Job drawing, mm, ordinate dimensions from the low corner. One solid piece. A direction names the side the tool comes from. Round coordinates to 2 decimals unless told otherwise and drop trailing zeros. Loops run counter-clockwise (first coordinate to the right, second up) from the corner with the lowest first, then second, coordinate; pieces in that order, holes last. Notation, with made-up numbers: M 55,-38 L 106,-38 A20 ccw 106,-12 Z; hole C 62.25,63 d4. An arc over 180 degrees is marked long. Put each result on its own line as item: value. Start each with the question number.
1) Slice it at C-C on y = 45. Give the cut face in (x, z) (1 decimal).
2) Slice it at D-D on x = 25.5. Give the cut face in (y, z).
3) Slice it at B-B on z = 28.5. Give the cut face in (x, y).
4) Probe line 1 along X through (y, z) = (35.5, 33); line 2 along Y through (x, z) = (3, 19); line 3 along X through (y, z) = (21, 18.5). List the from-to ranges inside material, lowest first.
5) Which spindle directions (+Z, -Z, +X, -X, +Y, -Y) get a long thin tool onto all of the face, cutting with end or side? Do the marked faces 4 and 5. Say none if no direction does.
6) Pull direction X, two halves, no side cores. Call the marked faces 1, 2 and 3: +X half, -X half, draft (parallel to the pull), parting line (faces both ways), or undercut.
7) Drop flat-ended pins along their axis: pin 1 Ø4 at (x, z) = (25.5, 37.5) entering from +Y; pin 2 Ø17.5 at (y, z) = (18, 36) entering from -X. Give the stop position or say it passes through.
8) Slice it at A-A on y = 12. Give the cut face in (x, z).
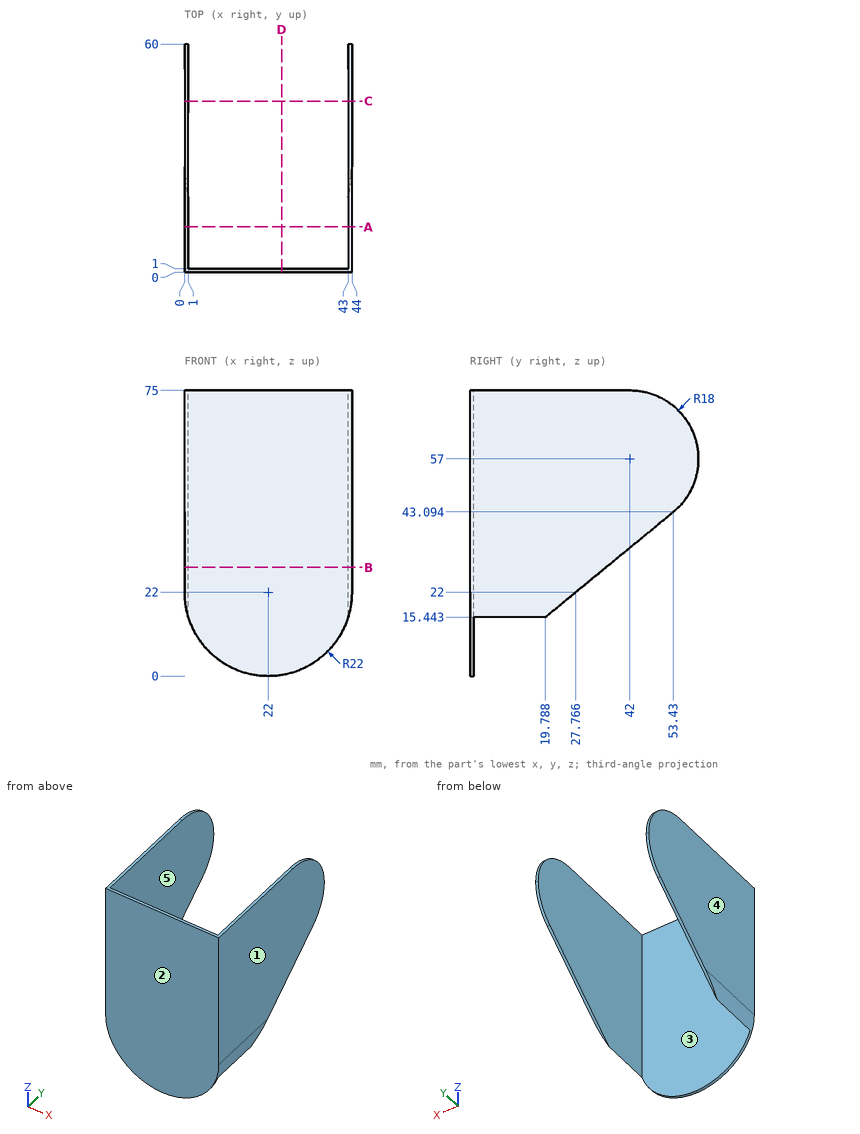
Recorded:
1. outline: M 0,36.2 L 1,36.2 L 1,74.7 L 0,74.7 Z; M 43,36.2 L 44,36.2 L 44,74.7 L 43,74.7 Z
2. outline: M 0,0.28 L 1,0.28 L 1,75 L 0,75 Z
3. outline: M 0,0 L 44,0 L 44,35.67 L 43,35.67 L 43,1 L 1,1 L 1,35.67 L 0,35.67 Z
4. line 1: x = 0 to 1, 43 to 44
4. line 2: y = 0 to 1
4. line 3: x = 0.28 to 1, 43 to 43.72
5. face 4: +Z, -Z, -X, +Y, -Y
5. face 5: +Z, -Z, +Y
6. face 1: +X half
6. face 2: draft
6. face 3: undercut
7. pin 1: stops at y = 1
7. pin 2: stops at x = 0
8. outline: M 0,22 A22 ccw 1,15.44 L 1,75 L 0,75 Z; M 43,15.44 A22 ccw 44,22 L 44,75 L 43,75 Z
